Check sheet for the modelled part. Datum: model origin and axes. Units: mm. Face numbers are marked on the shaded views. Round coordinates to 2 decimals unless told otherwise and drop trailing zeros. Write each loop counter-clockwise with the first axis right and the second up, starting at its lowest first coordinate (ties: lowest second). Pieces come first, ordered by that corner, then holes.
Autodesk Inventor part; units mm, degrees
ref_plane "YZ Plane" through (0, 0, 0) normal (1, 0, 0) x (0, 1, 0)
ref_plane "XZ Plane" through (0, 0, 0) normal (0, 1, 0) x (-1, 0, 0)
ref_plane "XY Plane" through (0, 0, 0) normal (0, 0, 1) x (1, 0, 0)
sketch "Sketch1" plane through (0, 0, 0) normal (0, 1, 0) x (-1, 0, 0)
  line L0 (0, 0) -> (112, 0)
  line L1 (112, 0) -> (112, 40)
  line L2 (112, 40) -> (0, 40)
  line L3 (0, 40) -> (0, 0)
  circle A0 centre (9.4996, 20) radius 5
  circle A1 centre (102.489, 20) radius 5
  dimension "d0" = 112
  dimension "d1" = 40
  dimension "d4" = 10
  dimension "d5" = 10
  dimension "d18" = 92.9894
  dimension "d19" = 9.4996
  dimension "d22" = 9.511
  dimension "d23" = 40
  dimension "d24" = 20
extrude "Extrusion1" add sketch "Sketch1" along normal blind 8
sketch "Sketch2" plane through (0, 8, 0) normal (0, 1, 0) x (1, 0, 0)
  circle A0 centre (-102.489, -20) radius 5
  circle A1 centre (-9.4996, -20) radius 5
  circle A2 centre (-102.489, -20) radius 9
  circle A3 centre (-9.4996, -20) radius 9
  dimension "d8" = 18
  dimension "d9" = 18
extrude "Extrusion2" add sketch "Sketch2" along normal blind 5
sketch "Sketch3" plane through (-112, 0, 0) normal (-1, 0, 0) x (0, 0, 1)
  line L0 (0, 0) -> (40, 0)
  line L1 (40, 0) -> (40, 8)
  line L2 (0, 8) -> (40, 8)
  line L3 (0, 0) -> (0, 8)
extrude "Extrusion3" add sketch "Sketch3" along normal blind 11
sketch "Sketch4" plane through (0, 0, 40) normal (1, 0, 0) x (0, 0, -1)
  line L0 (0, 0) -> (40, 0)
  line L1 (40, 0) -> (40, 8)
  line L2 (0, 8) -> (40, 8)
  line L3 (0, 0) -> (0, 8)
extrude "Extrusion4" add sketch "Sketch4" along normal blind 11
fillet "Fillet1" radius 1 13 edges at (-123, 4, 40) (-56, 0, 40) (-56, 0, 0) (-123, 0, 20) (11, 0, 20) (11, 4, 40) (11, 4, 0) (-56, 8, 0) (11, 8, 20) (-56, 8, 40) (-123, 8, 20) (-111.489, 13, 20) (-18.4996, 13, 20)
equation "\"d5\" = d4"
equation "\"d24\" = 0.5 * d23"
equation "\"d9\" = d8"
properties part number "CIM MountBase" material "Aluminum 6061, Welded"
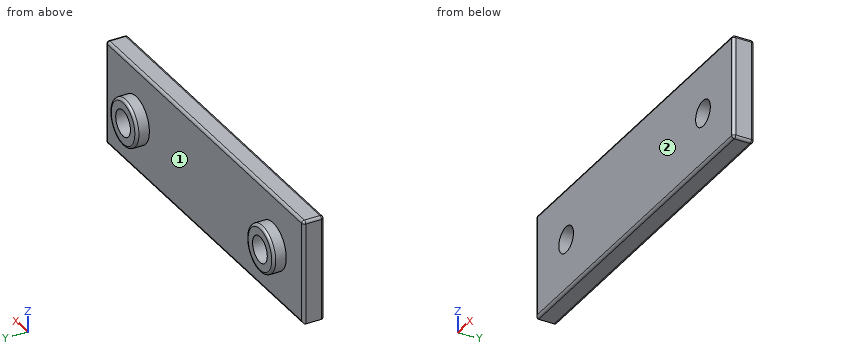
1. Sectioned sample at D-D, the plane z = 17.5. Give the number of separate pieces and of enclosed holes in the cut face, plus the area to 3 significant figures.
2. Sectioned sample at B-B, the plane x = -52. Enter the section's corners in (y, z), plus the area to 3 significant figures.
3. Sectioned sample at C-C, the plane z = 4.5. Enter the section's corners in (x, y).
4. Scan lines: line 1 along X through (y, z) = (6, 20); line 2 along X through (y, z) = (9.75, 20); line 3 along Y through (x, z) = (-29.5, 25). Record each from-to range of solid material in increasing order.
5. Release check for a two-part mould opening along X. For the marked faces 1 and 2 record: released by +X, released by -X, zero draft, split by the parting line, or undercut.
6. Go/stop test with flat-tipped pins: pin 1 (12 mm diameter, centred on x = -89, z = 24, fed in from +Y); pin 2 (1 mm diameter, centred on x = -99, y = 2, fed in from -Z); pin 3 (2 mm diameter, centred on x = -15, y = 9.5, fed in from +Z); pin 4 (12 mm diameter, centred on x = -79.5, z = 9.5, fed in from +Y). Record where each tip stops, or that it passes through.
7. Sectioned sample at A-A, the plane y = 2.25. Enter the section's corners in (x, z).
Computed values:
1. separate pieces: 3
1. enclosed holes: 0
1. area: 1,020 mm2
2. outline: (0, 1) arc R1 ccw to (1, 0) - (7, 0) arc R1 ccw to (8, 1) - (8, 39) arc R1 ccw to (7, 40) - (1, 40) arc R1 ccw to (0, 39) - close
2. area: 319 mm2
3. outline: (-123, 1) arc R1 ccw to (-122, 0) - (10, 0) arc R1 ccw to (11, 1) - (11, 7) arc R1 ccw to (10, 8) - (-122, 8) arc R1 ccw to (-123, 7) - close
4. line 1: x = -123 to -107.49, -97.49 to -14.5, -4.5 to 11
4. line 2: x = -111.49 to -107.49, -97.49 to -93.49, -18.5 to -14.5, -4.5 to -0.5
4. line 3: y = 0 to 8
5. face 1: undercut
5. face 2: zero draft
6. pin 1: stops at y = 13
6. pin 2: stops at z = 0
6. pin 3: stops at z = 27.79
6. pin 4: stops at y = 8
7. outline: (-123, 0) - (10, 0) arc R1 ccw to (11, 1) - (11, 39) arc R1 ccw to (10, 40) - (-122, 40) arc R1 ccw to (-123, 39) - close; hole circle Ø10 at (-102.49, 20); hole circle Ø10 at (-9.5, 20)
